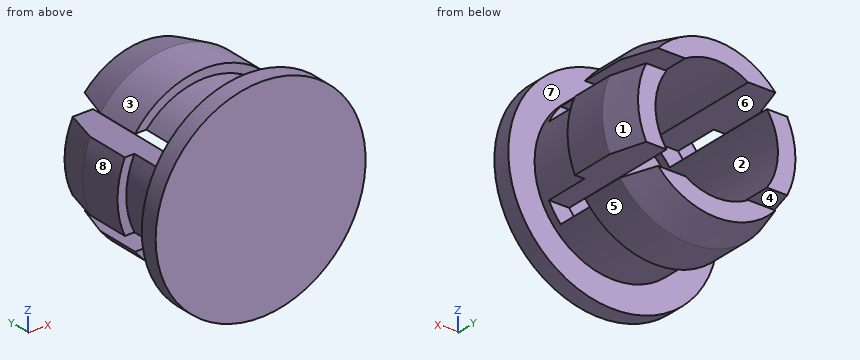
```python
from build123d import *

# Parameters (mm, degrees)
CROQUIS2_W            = 26
CROQUIS2_H            = 2
CORTAR_EXTRUIR1_DEPTH = 14


with BuildPart() as part:
    # Croquis1 → Revolución1 (revolve)
    with BuildSketch(Plane.XY):
        Polygon((-78.782252338, -15.637996222), (-90.782252338, -15.637996222), (-90.782252338, -13.637996222), (-87.782252338, -13.637996222), (-87.782252338, -7.637996222), (-88.782252338, -7.637996222), (-88.782252338, -2.637996222), (-87.782252338, 1.235955759), (-85.782252338, 1.235955759), (-85.782252338, -13.637996222), (-78.782252338, -13.637996222), align=None)
    revolve(axis=Axis((-78.782252338, -13.637996222, 0), (0, -1, 0)))

    # Croquis2 → Cortar-Extruir1 (cut)
    with BuildSketch(Plane(origin=(0, 1.235955759, 0), x_dir=(1, 0, 0), z_dir=(0, 1, 0))):
        with Locations((-78.782252338, -5)):
            Rectangle(CROQUIS2_W, CROQUIS2_H)
        with Locations((-78.782252338, 5)):
            Rectangle(CROQUIS2_W, CROQUIS2_H)
    extrude(amount=-CORTAR_EXTRUIR1_DEPTH, mode=Mode.SUBTRACT)


solid = part.part
```
Geometry: final body of the model. Coordinates: model frame, mm. Face numbers are marked on the shaded views. A direction names the side the tool comes from. Coordinates: 2 decimals unless noted, no trailing zeros. Write each loop counter-clockwise with the first axis right and the second up, starting at its lowest first coordinate (ties: lowest second). Pieces come first, ordered by that corner, then holes. Notation, with made-up numbers: M 70.5,89 L 78.5,89 A15 ccw 78.5,113 Z; hole C 33,-8.5 d6. An arc over 180 degrees is marked long. Use CSV: the item, a comma, the result in double quotes. Start each with the question number.
1. First-contact query: P1, Ø1.3, axis at x = -74, y = -8, coming from the +Z side; P2, Ø1, axis at x = -71, y = -9, coming from the +Z side; P3, Ø1.3, axis at x = -85, y = -7, coming from the -Z side. Flat tips, straight axial feed; report the tip coordinate or a pass-through.
2. Cut plane B-B on y = -6. Return the cut outline in (x, z).
3. Mould query, pull axis Z, two halves, no side actions, for the marked faces 1, 2, 3 and 4. Classes: pulls with the +Z half, pulls with the -Z half, needs draft (parallel to the pull), parting line crosses it, or undercut.
4. Reachability of the marked faces 5, 6, 7 and 8 from +Z, -Z, +X, -X, +Y, -Y: full face, straight path, thin tool, end or side. Return the list, or none.
5. Cut plane A-A on y = -10. Return the cut outline in (x, z), plus the area to 3 significant figures.
6. Cut plane C-C on z = 0. Return the cut outline in (x, y).
7. Ray query, probe 1 along Y at (x, z) = (-85.25, -9.25); probe 2 along Z at (x, y) = (-73.5, -8.5); probe 3 along X at (y, z) = (-2.75, 3.75). Return the intervals inside material, ascending.
Entries:
1,P1,"z = 9.06"
1,P2,"z = 4"
1,P3,"z = -8.31"
2,outline,"M -87.95,-4 L -84.53,-4 A7 cw -84.53,4 L -87.95,4 A10 ccw Z; M -86.78,-6 A10 ccw -70.78,-6 L -75.18,-6 A7 cw -82.39,-6 Z; M -86.78,6 L -82.39,6 A7 cw -75.18,6 L -70.78,6 A10 ccw Z; M -73.04,-4 L -69.62,-4 A10 ccw -69.62,4 L -73.04,4 A7 cw Z"
3,face 1,"parting line crosses it"
3,face 2,"undercut"
3,face 3,"pulls with the +Z half"
3,face 4,"undercut"
4,face 5,"-Z, +Y"
4,face 6,"+X, -X, +Y"
4,face 7,"none"
4,face 8,"-X, +Y"
5,outline,"M -86.84,-4 L -84.53,-4 A7 cw -84.53,4 L -86.84,4 A9 ccw Z; M -85.49,-6 A9 ccw -72.07,-6 L -75.18,-6 A7 cw -82.39,-6 Z; M -85.49,6 L -82.39,6 A7 cw -75.18,6 L -72.07,6 A9 ccw Z; M -73.04,-4 L -70.72,-4 A9 ccw -70.72,4 L -73.04,4 A7 cw Z"
5,area,"79.5 mm²"
6,outline,"M -90.78,-15.64 L -66.78,-15.64 L -66.78,-13.64 L -69.78,-13.64 L -69.78,-7.64 L -68.78,-7.64 L -68.78,-2.64 L -69.78,1.24 L -71.78,1.24 L -71.78,-13.64 L -85.78,-13.64 L -85.78,1.24 L -87.78,1.24 L -88.78,-2.64 L -88.78,-7.64 L -87.78,-7.64 L -87.78,-13.64 L -90.78,-13.64 Z"
7,probe 1,"-15.64 to -13.64"
7,probe 2,"-7.29 to -6, 6 to 7.29"
7,probe 3,"-88.05 to -84.69, -72.87 to -69.51"
